from build123d import *

# Parameters (mm, degrees)
PAD_DEPTH       = 7
SKETCH006_W     = 14
SKETCH006_H     = 14
PAD002_DEPTH    = 3
POCKET004_DEPTH = 2
SKETCH008_R     = 0.9
POCKET005_DEPTH = 1.001
FILLET001_R     = 1.5


with BuildPart() as clamp_unit001:
    # Sketch → Pad (new body, symmetric)
    with BuildSketch(Plane.XZ):
        Polygon((-2.6, 3.8), (4.2, 3.8), (4.2, 0), (2.6, 0), (2.6, 2.6), (-2.6, 2.6), (-2.6, 0), (-4.2, 0), (-4.2, 3.8), align=None)
    extrude(amount=PAD_DEPTH, both=True)


with BuildPart() as obj1:
    # Sketch006 → Pad002 (new body)
    with BuildSketch(Plane.XY):
        Rectangle(SKETCH006_W, SKETCH006_H)
    extrude(amount=PAD002_DEPTH)

    # Sketch007 → Pocket004 (cut)
    with BuildSketch(Plane.XY.offset(3)):
        with BuildLine():
            Line((-3, 7), (-3, 4.963869))
            ThreePointArc((-3, 4.963869), (-5.8, 0), (-3, -4.963869))
            Line((-3, -7), (-3, -4.963869))
            Line((3, -7), (-3, -7))
            Line((3, -4.963869), (3, -7))
            ThreePointArc((3, -4.963869), (5.8, 0), (3, 4.963869))
            Line((3, 7), (3, 4.963869))
            Line((-3, 7), (3, 7))
        make_face()
    extrude(amount=-POCKET004_DEPTH, mode=Mode.SUBTRACT)

    # Sketch008 → Pocket005 (cut, through all)
    with BuildSketch(Plane.XY.offset(1)):
        Circle(SKETCH008_R)
    extrude(amount=-POCKET005_DEPTH, mode=Mode.SUBTRACT)


with BuildPart() as obj1_1:
    # Clone placement: moved
    add(obj1.part.moved(Location((-11.2, 0, 0))))


with BuildPart() as obj2:
    # Clone004 base: copy of obj1
    add(obj1_1.part)


with BuildPart() as obj2_1:
    # Clone004 placement: moved
    add(obj2.part.moved(Location((22.4, 0, 0))))


with BuildPart() as clone_of_wire_holder_double:
    # Fusion001 base: copy of obj1
    add(obj1_1.part)

    # Fusion001: union clamp-unit001, obj2
    add(clamp_unit001.part)
    add(obj2_1.part)

    # Fillet001
    fillet001_edges = [clone_of_wire_holder_double.edges().sort_by_distance(p)[0] for p in [
        (-18.2, 7, 1.5),
        (18.2, 7, 1.5),
        (-18.2, -7, 1.5),
        (18.2, -7, 1.5),
    ]]
    fillet(fillet001_edges, radius=FILLET001_R)


with BuildPart() as clone_of_wire_holder_double_1:
    # Clone007 placement: moved
    add(clone_of_wire_holder_double.part.moved(Location((35.472096, 29.030871, 0))))


with BuildPart() as clone_of_wire_holder_double_2:
    # Clone001004 placement: moved
    add(clone_of_wire_holder_double_1.part.moved(Location((-23.02183, -12.928266, 39))))


solid = clone_of_wire_holder_double_2.part
Read the model definition and answer for the solid it produces. Units are mm, in the model's axes. A direction names the side the tool comes from. Round coordinates to 2 decimals unless told otherwise and drop trailing zeros. Order: outer loops, then holes, each group sorted by start corner. A loop starts at its lowest first (then second) coordinate and runs counter-clockwise, first axis right, second up. Notation, with made-up numbers: (16, 4) - (42, 4) arc R11 cw to (42, 24) - close; hole circle Ø10 at (72.25, -1). An arc over 180 degrees is marked (long way). Use one line per item in the form item = value. Start each with the question number.
(1) Flat-ended cylindrical pins translate along their axes: pin 1 Ø1.2 at (x, y) = (19.5, 15.5) entering from +Z; pin 2 Ø8 at (x, y) = (3, 19) entering from +Z; pin 3 Ø1.6 at (y, z) = (22.5, 40.5) entering from -X. Find the tip coordinate at first contact, or state that the pin passes through.
(2) Determine the mould class of faces 1 (the face through (15.05, 16, 40)), 2 (the face through (-5.3, 9.53, 40.52)), 3 (the face through (24.066, 15.304, 39.507)) for opening direction Y: +Y half, -Y half, draft (parallel to the pull), parting line (faces both ways), or undercut.
(3) The part is cut by section C-C (y = 13). Give the vertices of the cut face in (x, z).
(4) The part is cut by section D-D (x = 11.5). Give the vertices of the cut face in (y, z).
(5) The part is cut by section A-A (z = 40.7). Give the vertices of the cut face in (x, y), then the cut area to 3 significant figures.
(6) Find the intervals of material crossed by line 1 along X through (y, z) = (21.75, 41); line 2 along X through (y, z) = (11, 40.4); line 3 along X through (y, z) = (12.5, 39.7), in increasing order. Write a range as from..to.
(7) The part is cut by section B-B (x = 1). Give the vertices of the cut face in (y, z).
(8) For faces 4 (the face through (0, 16, 40)), 5 (the face through (20.65, 10, 41)), 6 (the face through (30.65, 16, 40)), 7 (the face through (12, 16, 41.6)), 8 (the face through (30.2, 9.53, 40.52)), determine the directions among +Z, -Z, +X, -X, +Y, -Y from which every point of the face is accessible in a straight line to the end or side of a thin tool.
Checked values:
q1.pin_1 = 40
q1.pin_2 = 42
q1.pin_3 = -5.75
q2.face_1 = draft
q2.face_2 = -Y half
q2.face_3 = undercut
q3.outline = (-5.75, 39) - (9.85, 39) - (9.85, 41.6) - (15.05, 41.6) - (15.05, 39) - (30.65, 39) - (30.65, 42) - (28.55, 42) - (28.55, 40) - (18.75, 40) - (18.75, 42) - (16.65, 42) - (16.65, 42.8) - (8.25, 42.8) - (8.25, 42) - (6.15, 42) - (6.15, 40) - (-3.65, 40) - (-3.65, 42) - (-5.75, 42) - close
q4.outline = (9.1, 41.6) - (23.1, 41.6) - (23.1, 42.8) - (9.1, 42.8) - close
q5.outline = (-5.75, 10.6) arc R1.5 ccw to (-4.25, 9.1) - (-1.75, 9.1) - (-1.75, 11.14) arc R5.8 cw to (-1.75, 21.07) - (-1.75, 23.1) - (-4.25, 23.1) arc R1.5 ccw to (-5.75, 21.6) - close; (4.25, 9.1) - (9.85, 9.1) - (9.85, 23.1) - (4.25, 23.1) - (4.25, 21.07) arc R5.8 cw to (4.25, 11.14) - close; (15.05, 9.1) - (20.65, 9.1) - (20.65, 11.14) arc R5.8 cw to (20.65, 21.07) - (20.65, 23.1) - (15.05, 23.1) - close; (26.65, 9.1) - (29.15, 9.1) arc R1.5 ccw to (30.65, 10.6) - (30.65, 21.6) arc R1.5 ccw to (29.15, 23.1) - (26.65, 23.1) - (26.65, 21.07) arc R5.8 cw to (26.65, 11.14) - close
q5.area = 188 mm^2
q6.line_1 = -5.74..-1.75, 4.25..9.85, 15.05..20.65, 26.65..30.64
q6.line_2 = -5.75..-1.75, 4.25..9.85, 15.05..20.65, 26.65..30.65
q6.line_3 = -5.75..9.85, 15.05..30.65
q7.outline = (9.1, 39) - (15.24, 39) - (15.24, 40) - (9.1, 40) - close; (16.97, 39) - (23.1, 39) - (23.1, 40) - (16.97, 40) - close
q8.face_4 = +Z
q8.face_5 = +Z, +Y, -Y
q8.face_6 = +Z, -Z, +X, +Y, -Y
q8.face_7 = -Z, +Y, -Y
q8.face_8 = +Z, -Z, +X, -Y
